Check sheet for the modelled part. Datum: model origin and axes. Units: mm. A direction names the side the tool comes from. Round coordinates to 2 decimals unless told otherwise and drop trailing zeros. Loops run counter-clockwise (first coordinate to the right, second up) from the corner with the lowest first, then second, coordinate; pieces in that order, holes last. Notation, with made-up numbers: M -27.5,67 L -1.5,67 A31 ccw -1.5,103 Z; hole C 4.25,27.5 d9. An arc over 180 degrees is marked long. Write item = value, one per line. Start each with the question number.
(1) Scan lines: L1, parallel to Z at x = -3.5, y = 3; L2, parallel to Z at x = -7.5, y = 1.45; L3, parallel to Z at x = -6.75, y = 1. Record each from-to range of solid material in increasing order. Write a range as from..to.
(2) Cross-section at B-B on x = -3.5. Record the boundary of the cut face in (y, z), plus the area to 3 significant figures.
(3) Cross-section at C-C on x = -8. Record the boundary of the cut face in (y, z).
(4) Cross-section at D-D on y = 0.85. Record the boundary of the cut face in (x, z).
(5) Set-up check for faces 5 (the face through (1.603, 3, 11)), 6 (the face through (-9.796, 0.842, 12.829)), 7 (the face through (-4.577, 3, 11)): record each of +Z, -Z, +X, -X, +Y, -Y from which the full face is reachable in a straight line by a thin tool's end or side.
(6) Mould release check, pull along Z, two halves, no side actions. Record for faces 1 (the face through (-2, 2, -12.22)), 2 (the face through (-1, 3, -7.87)), 3 (the face through (-1, 0, 0)), 4 (the face through (4.01, 0.82, 11.55)): pulls with the +Z half, pulls with the -Z half, needs draft (parallel to the pull), parting line crosses it, or undercut.
(7) Go/stop test with flat-tipped pins: P1, Ø1.7, axis at y = 3.5, z = 11.5, coming from the -X side; P2, Ø1, axis at y = 3.5, z = -9.5, coming from the +X side; P3, Ø1, axis at x = 0, z = 4, coming from the +Y side. Record where each tip stops, or that it passes through.
(8) Cross-section at A-A on y = 2.05. Record the boundary of the cut face in (x, z), plus the area to 3 significant figures.
from build123d import *

# Parameters (mm, degrees)
SKETCH1_W           = 17.82
SKETCH1_H           = 25.62
BOSS_EXTRUDE1_DEPTH = 1.66
SKETCH2_W           = 6.18
SKETCH2_H           = 4.35
BOSS_EXTRUDE2_DEPTH = 5
FILLET1_R           = 2
HOLE1_D             = 2.5


with BuildPart() as part:
    # Sketch1 → Boss-Extrude1 (new body)
    with BuildSketch(Plane(origin=(0, 0, 0), x_dir=(1, 0, 0), z_dir=(0, 1, 0))):
        with Locations((-1.487037037, -0.58962963)):
            Rectangle(SKETCH1_W, SKETCH1_H)
    extrude(amount=BOSS_EXTRUDE1_DEPTH)

    # Sketch2 → Boss-Extrude2 (add)
    with BuildSketch(Plane(origin=(0, 0, 0), x_dir=(-1, 0, 0), z_dir=(0, -1, 0))):
        with Locations((1.487037037, -11.22462963)):
            Rectangle(SKETCH2_W, SKETCH2_H)
        with Locations((1.487037037, 10.04537037)):
            Rectangle(SKETCH2_W, SKETCH2_H)
    extrude(amount=-BOSS_EXTRUDE2_DEPTH)

    # Fillet1
    fillet1_edges = [part.edges().sort_by_distance(p)[0] for p in [
        (-10.397037037, 0.83, -12.22037037),
        (7.422962963, 0.83, -12.22037037),
        (7.422962963, 0.83, 13.39962963),
        (-10.397037037, 0.83, 13.39962963),
    ]]
    fillet(fillet1_edges, radius=FILLET1_R)

    # Hole1 (through all)
    with Locations(Plane(origin=(0, 1.66, 0), x_dir=(1, 0, 0), z_dir=(0, 1, 0))):
        with Locations((4.591727838, -10.44356219), (-7.580024265, -10.44356219), (-7.580024265, 8.909603349), (4.591727838, 8.909603349)):
            Hole(HOLE1_D / 2)


solid = part.part
Result:
q1.L1 = -12.22..-7.87, 9.05..13.4
q1.L2 = -12.22..-10.16, -7.66..9.2, 11.69..13.4
q1.L3 = -12.22..-9.84, -7.97..9.51, 11.38..13.4
q2.outline = M 0,-12.22 L 5,-12.22 L 5,-7.87 L 1.66,-7.87 L 1.66,9.05 L 5,9.05 L 5,13.4 L 0,13.4 Z
q2.area = 71.6 mm^2
q3.outline = M 0,-12.22 L 1.66,-12.22 L 1.66,-10.09 L 0,-10.09 Z; M 0,-7.73 L 1.66,-7.73 L 1.66,9.27 L 0,9.27 Z; M 0,11.62 L 1.66,11.62 L 1.66,13.4 L 0,13.4 Z
q4.outline = M -10.4,-10.22 A2 ccw -8.4,-12.22 L 5.42,-12.22 A2 ccw 7.42,-10.22 L 7.42,11.4 A2 ccw 5.42,13.4 L -8.4,13.4 A2 ccw -10.4,11.4 Z; hole C -7.58,-8.91 d2.5; hole C -7.58,10.44 d2.5; hole C 4.59,-8.91 d2.5; hole C 4.59,10.44 d2.5
q5.face_5 = +Z, -Z, +X, +Y
q5.face_6 = +Z, -X, +Y, -Y
q5.face_7 = +Z, -Z, -X, +Y
q6.face_1 = pulls with the -Z half
q6.face_2 = undercut
q6.face_3 = needs draft
q6.face_4 = undercut
q7.P1 = -4.58
q7.P2 = 1.6
q7.P3 = 1.66
q8.outline = M -4.58,-12.22 L 1.6,-12.22 L 1.6,-7.87 L -4.58,-7.87 Z; M -4.58,9.05 L 1.6,9.05 L 1.6,13.4 L -4.58,13.4 Z
q8.area = 53.8 mm^2
